Build history of the part. All positions in model axes, mm. A direction names the side the tool comes from. Round coordinates to 2 decimals unless told otherwise and drop trailing zeros. Order: outer loops, then holes, each group sorted by start corner. A loop starts at its lowest first (then second) coordinate and runs counter-clockwise, first axis right, second up. Notation, with made-up numbers: M -6.5,34.25 L 12.5,34.25 A15 ccw 12.5,45.25 Z; hole C 1,32.5 d7. An arc over 180 degrees is marked long. Use CSV: the item, a comma, the result in double quotes.
Autodesk Inventor part; units mm, degrees
ref_plane "YZ Plane" through (0, 0, 0) normal (1, 0, 0) x (0, 1, 0)
ref_plane "XZ Plane" through (0, 0, 0) normal (0, 1, 0) x (-1, 0, 0)
ref_plane "XY Plane" through (0, 0, 0) normal (0, 0, 1) x (1, 0, 0)
sketch "スケッチ1" plane through (0, 0, 0) normal (0, 0, 1) x (1, 0, 0)
  arc A0 (-2, 1.8875) -> (-2, -1.8875) centre (0, 0) ccw
  line L0 (-2, 1.8875) -> (2, 1.8875)
  line L1 (2, -1.8875) -> (-2, -1.8875)
  arc A1 (2, -1.8875) -> (2, 1.8875) centre (0, 0) ccw
  circle A2 centre (0, 0) radius 3.5
  point P0 (0, 0)
  dimension "d0" = 7
extrude "押し出し1" add sketch "スケッチ1" against normal blind 8
sketch "スケッチ2" plane through (0, 0, 0) normal (0, 0, 1) x (1, 0, 0)
  circle A0 centre (0, 0) radius 3.5
  circle A1 centre (0, 0) radius 4
  point P0 (0, 0)
  dimension "d3" = 8
extrude "押し出し2" add sketch "スケッチ2" along normal blind 5 contours A0 | A1
sketch "スケッチ3" plane through (0, 0, 5) normal (0, 0, 1) x (1, 0, 0)
  circle A0 centre (0, 0) radius 3
  dimension "d6" = 6
extrude "押し出し3" add sketch "スケッチ3" along normal blind 10
properties part number "カップリング"
(1) Cut at D-D, the plane z = 13.25. Give the cut face in (x, y).
Answer block:
outline,"C 0,0 d6"
(2) Drop flat-ended pins along their axis: pin 1 (1.9 mm diameter, centred on x = -1, y = -0.5, fed in from -Z); pin 2 (4.5 mm diameter, centred on x = 0.5, z = -4, fed in from +Y); pin 3 (3 mm diameter, centred on x = 2.5, z = 3, fed in from -Y). Give the stop position or say it passes through.
Answer block:
pin 1,"stops at z = 0"
pin 2,"stops at y = 3.5"
pin 3,"stops at y = -3.87"
(3) Cut at B-B, the plane x = 0. Give the cut face in (y, z), and give its area (3 significant figures).
Answer block:
outline,"M -4,0 L -3.5,0 L -3.5,-8 L -1.89,-8 L -1.89,0 L 1.89,0 L 1.89,-8 L 3.5,-8 L 3.5,0 L 4,0 L 4,5 L 3,5 L 3,15 L -3,15 L -3,5 L -4,5 Z"
area,"126 mm²"
(4) Wall check: line 1 (Z direction, x = 1, y = 3.25); line 2 (Z direction, x = 1, y = 1); line 3 (Y direction, x = -0.5, z = -2.5). Give the ranges that are in metal, low to high. Write a range as from..to.
Answer block:
line 1,"z = -8..5"
line 2,"z = 0..15"
line 3,"y = -3.46..-1.89, 1.89..3.46"
(5) Cut at C-C, the plane z = -6.25. Give the cut face in (x, y), and give its area (3 significant figures).
Answer block:
outline,"C 0,0 d7; hole M -2,-1.89 L 2,-1.89 A2.75 ccw 2,1.89 L -2,1.89 A2.75 ccw Z"
area,"19.5 mm²"
(6) Two-plate mould, pull along X, no slides. Class faces 4 (the face through (0, 1.888, -4)), 5 (the face through (0, -2.3, -8)), 6 (the face through (-3, 0, 10)): released by +X, released by -X, zero draft, split by the parting line, or undercut.
Answer block:
face 4,"undercut"
face 5,"zero draft"
face 6,"split by the parting line"
(7) Cut at A-A, the plane y = 0. Give the cut face in (x, z), and give its area (3 significant figures).
Answer block:
outline,"M -4,0 L -3.5,0 L -3.5,-8 L -2.75,-8 L -2.75,0 L 2.75,0 L 2.75,-8 L 3.5,-8 L 3.5,0 L 4,0 L 4,5 L 3,5 L 3,15 L -3,15 L -3,5 L -4,5 Z"
area,"112 mm²"
(8) Tool access for faces 1 (the face through (-0.867, 3.905, 2.465)), 2 (the face through (0, 0, 0)), 3 (the face through (1, 3, 5)): list every direction of +Z, -Z, +X, -X, +Y, -Y with a clear straight run to the whole face (end or side of a thin tool).
Answer block:
face 1,"+Z, -Z"
face 2,"-Z"
face 3,"+Z"
